Design review of the part built by this model. Coordinates are the model's own, in mm. A direction names the side the tool comes from. Round coordinates to 2 decimals unless told otherwise and drop trailing zeros. Write each loop counter-clockwise with the first axis right and the second up, starting at its lowest first coordinate (ties: lowest second). Pieces come first, ordered by that corner, then holes. Notation, with made-up numbers: M -15.75,-21.5 L 42.25,-21.5 A6 cw 42.25,-14.5 Z; hole C -7,-11.75 d1. An arc over 180 degrees is marked long. One line per question, with ' | ' between items. Start each with the question number.
Item 1: Machinability: for faces 4 (the face through (-17, 35, -4)), 5 (the face through (49.465, 3.905, 0.867)), 6 (the face through (-25, 35, 0)), which of the approach directions +Z, -Z, +X, -X, +Y, -Y give a long, thin tool a straight path to every point of the face, cutting with its end or side? Answer none if there is none.
Item 2: Add section A-A, the plane y = 25. State the section outline as (x, z) points, and give its area (3 significant figures).
Item 3: Add section C-C, the plane y = 0. State the section outline as (x, z) points.
Item 4: For L1, parallel to X at y = 25, z = 1; L2, parallel to X at y = 1, z = 3.25; L3, parallel to Z at x = 21, y = 45.5, list the stretches that pass through material, from the lowest coordinate up.
Item 5: Insertion check: pin 1 Ø8 at (x, y) = (-17, 39.5) entering from +Z; pin 2 Ø2.5 at (y, z) = (31, 1.5) entering from +X; pin 3 Ø1.5 at (y, z) = (12.5, -3) entering from +X; pin 4 Ø5 at (x, y) = (22.5, 17) entering from +Z. Each pin has a flat end and moves straight along its axis. Give the tip position at first contact, or say it passes through.
Item 6: Add section D-D, the plane x = 44. State the section outline as (y, z) points, and give its area (3 significant figures).
Item 7: Draft analysis for pull direction X (two halves, no side actions). For faces 1 (the face through (-47, 0, 0)), 2 (the face through (52, 2, -2)), 3 (the face through (-29, 35, 0)), state which applies: released by +X, released by -X, zero draft, split by the parting line, or undercut.
Autodesk Inventor part; units mm, degrees
ref_plane "YZ Plane" through (0, 0, 0) normal (1, 0, 0) x (0, 1, 0)
ref_plane "XZ Plane" through (0, 0, 0) normal (0, 1, 0) x (-1, 0, 0)
ref_plane "XY Plane" through (0, 0, 0) normal (0, 0, 1) x (1, 0, 0)
sketch "スケッチ1" plane through (0, 0, 0) normal (0, 0, 1) x (1, 0, 0)
  line L0 (47, -15.5) -> (-47, -15.5)
  line L1 (-47, -15.5) -> (-47, 15.5)
  line L2 (-47, 15.5) -> (47, 15.5)
  line L3 (47, 15.5) -> (47, -15.5)
  line L4 (47, -15.5) -> (-47, 15.5) construction
  line L5 (-47, -15.5) -> (47, 15.5) construction
  point P0 (0, 0)
  dimension "d0" = 94
  dimension "d1" = 31
extrude "押し出し1" add sketch "スケッチ1" along normal mid plane 10
sketch "スケッチ2" plane through (47, -15.5, 5) normal (1, 0, 0) x (0, 0, -1)
  circle A0 centre (5, 15.5) radius 4
  dimension "d4" = 8
extrude "押し出し2" add sketch "スケッチ2" along normal blind 5
sketch "スケッチ3" plane through (52, 0, 0) normal (1, 0, 0) x (0, 0, -1)
  circle A0 centre (0, 0) radius 2.5
  dimension "d7" = 5
extrude "押し出し3" add sketch "スケッチ3" along normal blind 10
fillet "フィレット1" radius 0.5 12 edges at (0, 15.5, 5) (47, 0, 5) (47, 15.5, 0) (47, -15.5, 0) (0, -15.5, 5) (0, 15.5, -5) (0, -15.5, -5) (47, 0, -5) (-47, 0, 5) (-47, 15.5, 0) (-47, 0, -5) (-47, -15.5, 0)
sketch "スケッチ4" plane through (-46.5, 15.5, -4.5) normal (0, 1, 0) x (1, 0, 0)
  line L0 (1.5, -0.5) -> (17.5, -0.5)
  line L1 (17.5, -0.5) -> (17.5, -8.5)
  line L2 (17.5, -8.5) -> (1.5, -8.5)
  line L3 (1.5, -8.5) -> (1.5, -0.5)
  line L4 (1.5, -0.5) -> (17.5, -8.5) construction
  line L5 (17.5, -0.5) -> (1.5, -8.5) construction
  line L6 (-0.5, 0) -> (-0.5, -9)
  point P0 (46.5, -4.5)
  point P1 (9.5, -4.5)
  point P2 (9.5, -4.5)
  dimension "d11" = 8
  dimension "d12" = 16
  dimension "d13" = 10
extrude "押し出し4" add sketch "スケッチ4" along normal blind 40
pattern_linear "矩形状パターン1" count 4 spacing 20 along (1, 0, 0) of "押し出し4"
properties part number "U3H-FC03BBK" material "ABS プラスチック"
Computed values:
1) face 4: -Z, +X, -X, +Y | face 5: +X | face 6: +Z, -Z, +Y
2) outline: M -45,-4 L -29,-4 L -29,4 L -45,4 Z; M -25,-4 L -9,-4 L -9,4 L -25,4 Z; M -5,-4 L 11,-4 L 11,4 L -5,4 Z; M 15,-4 L 31,-4 L 31,4 L 15,4 Z | area: 512 mm^2
3) outline: M -47,-4.5 A0.5 ccw -46.5,-5 L 46.5,-5 A0.5 ccw 47,-4.5 L 47,-4 L 52,-4 L 52,-2.5 L 62,-2.5 L 62,2.5 L 52,2.5 L 52,4 L 47,4 L 47,4.5 A0.5 ccw 46.5,5 L -46.5,5 A0.5 ccw -47,4.5 Z
4) L1: x = -45 to -29, -25 to -9, -5 to 11, 15 to 31 | L2: x = -47 to 52 | L3: z = -4 to 4
5) pin 1: stops at z = 4 | pin 2: stops at x = 31 | pin 3: stops at x = 47 | pin 4: stops at z = 5
6) outline: M -15.5,-4.5 A0.5 ccw -15,-5 L 15,-5 A0.5 ccw 15.5,-4.5 L 15.5,4.5 A0.5 ccw 15,5 L -15,5 A0.5 ccw -15.5,4.5 Z | area: 310 mm^2
7) face 1: released by -X | face 2: released by +X | face 3: undercut
